Input: part model. Units: mm. Frame: model coordinates. A direction names the side the tool comes from. Coordinates: 2 decimals unless noted, no trailing zeros. Write each loop counter-clockwise with the first axis right and the second up, starting at its lowest first coordinate (ties: lowest second). Pieces come first, ordered by that corner, then holes.
1) Section query A-A (z = -10.5). Output: boundary loops of the cut face in (x, y), then the cut area to 3 significant figures.
2) Section query B-B (x = 19.5). Output: boundary loops of the cut face in (y, z), then the cut area to 3 significant figures.
3) Section query C-C (y = 5). Output: boundary loops of the cut face in (x, z).
4) Pin query (flat end, axial travel): pin 1 Ø10 at (x, z) = (-28, 28.5) entering from -Y; pin 2 Ø7.5 at (x, y) = (8.5, 41) entering from +Z; pin 3 Ø2 at (x, y) = (-45, 12.5) entering from -Z; pin 4 Ø18 at (x, y) = (-47.7, -4.97) entering from -Z. Return the tip coordinate at first contact, or that it passes through.
5) Section query D-D (z = 15). Output: boundary loops of the cut face in (x, y), then the cut area to 3 significant figures.
6) Set-up query: faces 1 (the flat face through (1, 25.032, 30)), 2 (the flat face through (1, -5, 40)), 3 (the flat face through (1, -5, 0)). Return all of +Z, -Z, +X, -X, +Y, -Y with unobstructed straight access to the full face (end or side cutting, diameter ignored); none if empty.
7) Line query: L1, parallel to Y at x = 57, z = -2; L2, parallel to X at y = -6, z = 28; L3, parallel to X at y = -12.5, z = 10. Output: solid intervals per line, ascending.
8) Draft query along Y for faces 4 (the flat face through (1, -34.968, 30)), 5 (the flat face through (1, -47, 20)), 6 (the cylindrical face through (37.317, -4.309, 19.72)). Return one class per face: pulls with the +Y half, pulls with the -Y half, needs draft (parallel to the pull), parting line crosses it, or undercut.
from build123d import *

# Parameters (mm, degrees)
F0_W     = 200
F0_H     = 60
F0_R     = 15
F1_DEPTH = 40
F2_W     = 200
F2_H     = 40
F3_DEPTH = 25
F4_W     = 200
F4_H     = 40
F5_DEPTH = 25


with BuildPart() as f1:
    # F0 (on Top) → F1 (new body)
    with BuildSketch(Plane.XY):
        with Locations((2.302447, -4.968402)):
            Rectangle(F0_W, F0_H)
        with Locations((-47.697553, -4.968402)):
            Circle(F0_R, mode=Mode.SUBTRACT)
        with Locations((52.302447, -4.968402)):
            Circle(F0_R, mode=Mode.SUBTRACT)
    extrude(amount=F1_DEPTH)

    # F2 (on face) → F3 (join)
    with BuildSketch(Plane.XZ.offset(34.968402)):
        with Locations((2.302447, 0)):
            Rectangle(F2_W, F2_H)
    extrude(amount=F3_DEPTH)

    # F4 (on face) → F5 (join)
    with BuildSketch(Plane(origin=(0, 25.031598, 0), x_dir=(-1, 0, 0), z_dir=(0, 1, 0))):
        with Locations((-2.302447, 0)):
            Rectangle(F4_W, F4_H)
    extrude(amount=F5_DEPTH)


solid = f1.part
Answer:
1. outline: (-97.7, -59.97) - (102.3, -59.97) - (102.3, -34.97) - (-97.7, -34.97) - close; (-97.7, 25.03) - (102.3, 25.03) - (102.3, 50.03) - (-97.7, 50.03) - close
1. area: 10,000 mm2
2. outline: (-59.97, -20) - (-34.97, -20) - (-34.97, 0) - (25.03, 0) - (25.03, -20) - (50.03, -20) - (50.03, 20) - (25.03, 20) - (25.03, 40) - (-34.97, 40) - (-34.97, 20) - (-59.97, 20) - close
2. area: 4,400 mm2
3. outline: (-97.7, 0) - (-58.91, 0) - (-58.91, 40) - (-97.7, 40) - close; (-36.49, 0) - (41.09, 0) - (41.09, 40) - (-36.49, 40) - close; (63.51, 0) - (102.3, 0) - (102.3, 40) - (63.51, 40) - close
4. pin 1: stops at y = -34.97
4. pin 2: stops at z = 20
4. pin 3: stops at z = 0
4. pin 4: passes through
5. outline: (-97.7, -59.97) - (102.3, -59.97) - (102.3, 50.03) - (-97.7, 50.03) - close; hole circle Ø30 at (-47.7, -4.97); hole circle Ø30 at (52.3, -4.97)
5. area: 20,600 mm2
6. face 1: +Z, +X, -X, +Y
6. face 2: +Z, +X, -X, +Y, -Y
6. face 3: -Z, +X, -X
7. L1: y = -59.97 to -34.97, 25.03 to 50.03
7. L2: x = -97.7 to -62.66, -32.73 to 37.34, 67.27 to 102.3
7. L3: x = -97.7 to -60.67, -34.73 to 39.33, 65.27 to 102.3
8. face 4: pulls with the -Y half
8. face 5: needs draft
8. face 6: undercut
